Geometry: final body of the model. Coordinates: model frame, mm. A direction names the side the tool comes from. Give positions to 0.01 mm unless a question says otherwise; leave off trailing zeros. Loops run counter-clockwise (first coordinate to the right, second up) from the corner with the lowest first, then second, coordinate; pieces in that order, holes last. Notation, with made-up numbers: M 65.5,57.5 L 109.5,57.5 A19 ccw 109.5,76.5 Z; hole C 82,54.25 d2. An arc over 180 degrees is marked long. Put each result on its own line as item: value.
```python
from build123d import *

# Parameters (mm, degrees)
F0_W      = 151.771664
F0_H      = 152.44925
F1_DEPTH  = 2.54
F2_W      = 133.218258
F2_H      = 132.201344
F3_DEPTH  = 2.54
F4_W      = 113.705158
F4_H      = 116.420522
F5_DEPTH  = 6.35
F6_W      = 94.709642
F6_H      = 95.752604
F7_DEPTH  = 6.35
F8_W      = 77.787876
F8_H      = 80.85847
F9_DEPTH  = 6.35
F10_W     = 63.117356
F10_H     = 65.164418
F11_DEPTH = 6.35
F12_W     = 48.859716
F12_H     = 52.300558
F13_DEPTH = 6.35
F14_W     = 37.017644
F14_H     = 37.017658
F15_DEPTH = 6.35
F16_W     = 23.323506
F16_H     = 24.019762
F17_DEPTH = 2.54
F18_W     = 16.055972
F18_H     = 16.134798
F19_DEPTH = 2.54
F20_W     = 9.981216
F20_H     = 9.746186
F21_DEPTH = 2.54


with BuildPart() as f1:
    # F0 (on Top) → F1 (new body)
    with BuildSketch(Plane.XY):
        Rectangle(F0_W, F0_H)
    extrude(amount=F1_DEPTH)

    # F2 (on face) → F3 (join)
    with BuildSketch(Plane.XY.offset(2.54)):
        Rectangle(F2_W, F2_H)
    extrude(amount=F3_DEPTH)

    # F4 (on face) → F5 (join)
    with BuildSketch(Plane.XY.offset(5.08)):
        Rectangle(F4_W, F4_H)
    extrude(amount=F5_DEPTH)

    # F6 (on face) → F7 (join)
    with BuildSketch(Plane.XY.offset(11.43)):
        Rectangle(F6_W, F6_H)
    extrude(amount=F7_DEPTH)

    # F8 (on face) → F9 (join)
    with BuildSketch(Plane.XY.offset(17.78)):
        Rectangle(F8_W, F8_H)
    extrude(amount=F9_DEPTH)

    # F10 (on face) → F11 (join)
    with BuildSketch(Plane.XY.offset(24.13)):
        Rectangle(F10_W, F10_H)
    extrude(amount=F11_DEPTH)

    # F12 (on face) → F13 (join)
    with BuildSketch(Plane.XY.offset(30.48)):
        Rectangle(F12_W, F12_H)
    extrude(amount=F13_DEPTH)

    # F14 (on face) → F15 (join)
    with BuildSketch(Plane.XY.offset(36.83)):
        Rectangle(F14_W, F14_H)
    extrude(amount=F15_DEPTH)

    # F16 (on face) → F17 (join)
    with BuildSketch(Plane.XY.offset(43.18)):
        Rectangle(F16_W, F16_H)
    extrude(amount=F17_DEPTH)

    # F18 (on face) → F19 (join)
    with BuildSketch(Plane.XY.offset(45.72)):
        Rectangle(F18_W, F18_H)
    extrude(amount=F19_DEPTH)

    # F20 (on face) → F21 (join)
    with BuildSketch(Plane.XY.offset(48.26)):
        Rectangle(F20_W, F20_H)
    extrude(amount=F21_DEPTH)


solid = f1.part
```
Item 1: Pin query (flat end, axial travel): pin 1 Ø3 at (y, z) = (10, 32.5) entering from +X; pin 2 Ø0.8 at (x, z) = (28, 3.5) entering from +Y; pin 3 Ø3 at (y, z) = (16, 20) entering from +X; pin 4 Ø4 at (x, y) = (-31, -29) entering from -Z. Return the tip coordinate at first contact, or that it passes through.
Output values:
pin 1: x = 24.43
pin 2: y = 66.1
pin 3: x = 38.89
pin 4: z = 0
Item 2: Line query: probe 1 along X at (y, z) = (-27, 24); probe 2 along Z at (x, y) = (-36, 52); probe 3 along Z at (x, y) = (22.5, 13). Output: solid intervals per line, ascending. Write a range as [from, to].
Output values:
probe 1: [-38.89, 38.89]
probe 2: [0, 11.43]
probe 3: [0, 36.83]
Item 3: Section D-D on y = 45.5. Output: boundary loops of the cut face in (x, z), then the cut area to 3 significant figures.
Output values:
outline: M -75.89,0 L 75.89,0 L 75.89,2.54 L 66.61,2.54 L 66.61,5.08 L 56.85,5.08 L 56.85,11.43 L 47.35,11.43 L 47.35,17.78 L -47.35,17.78 L -47.35,11.43 L -56.85,11.43 L -56.85,5.08 L -66.61,5.08 L -66.61,2.54 L -75.89,2.54 Z
area: 2,050 mm²
Item 4: Set-up query: faces 1 (the flat face through (-1, 47.876, 15)), 2 (the flat face through (-1, -40.429, 21)), 3 (the flat face through (56.853, -1, 8)). Return all of +Z, -Z, +X, -X, +Y, -Y with unobstructed straight access to the full face (end or side cutting, diameter ignored); none if empty.
Output values:
face 1: +Z, +X, -X, +Y
face 2: +Z, +X, -X, -Y
face 3: +Z, +X, +Y, -Y
Item 5: Section B-B on y = -30. Output: boundary loops of the cut face in (x, z), then the cut area to 3 significant figures.
Output values:
outline: M -75.89,0 L 75.89,0 L 75.89,2.54 L 66.61,2.54 L 66.61,5.08 L 56.85,5.08 L 56.85,11.43 L 47.35,11.43 L 47.35,17.78 L 38.89,17.78 L 38.89,24.13 L 31.56,24.13 L 31.56,30.48 L -31.56,30.48 L -31.56,24.13 L -38.89,24.13 L -38.89,17.78 L -47.35,17.78 L -47.35,11.43 L -56.85,11.43 L -56.85,5.08 L -66.61,5.08 L -66.61,2.54 L -75.89,2.54 Z
area: 2,940 mm²
Item 6: Section C-C on z = 35. Output: boundary loops of the cut face in (x, y).
Output values:
outline: M -24.43,-26.15 L 24.43,-26.15 L 24.43,26.15 L -24.43,26.15 Z
Item 7: Section A-A on x = 33.5. Output: boundary loops of the cut face in (y, z).
Output values:
outline: M -76.22,0 L 76.22,0 L 76.22,2.54 L 66.1,2.54 L 66.1,5.08 L 58.21,5.08 L 58.21,11.43 L 47.88,11.43 L 47.88,17.78 L 40.43,17.78 L 40.43,24.13 L -40.43,24.13 L -40.43,17.78 L -47.88,17.78 L -47.88,11.43 L -58.21,11.43 L -58.21,5.08 L -66.1,5.08 L -66.1,2.54 L -76.22,2.54 Z
